The listing builds one solid part. Answer for the finished solid, in the listing's coordinates (mm). A direction names the side the tool comes from. Round coordinates to 2 decimals unless told otherwise and drop trailing zeros.
(1) Find the intervals of material crossed by probe 1 along Z at (x, y) = (0, 3.5); probe 2 along X at (y, z) = (1.1, 0), in increasing order.
(2) For faces 5 (the face through (27.5, 3.9, -0.1)), 6 (the face through (15.05, 3.17, 23.61)), 7 (the face through (-15.79, 4.71, -20.97)), determine the directions among +Z, -Z, +X, -X, +Y, -Y from which every point of the face is accessible in a straight line to the end or side of a thin tool.
(3) Each of these flat-tipped pins is pushed along its axis until it touches: pin 1 Ø2 at (x, z) = (2, -27) entering from +Y; pin 2 Ø1 at (x, z) = (-17.5, 6.5) entering from +Y; pin 3 Ø1 at (x, y) = (11.5, 4) entering from -Z. Where does it stop, or does it pass through?
(4) The mould has two halves that part along Y. Classify faces 1 (the face through (16, 4, 21)), 2 (the face through (-0.1, 3.9, -27.5)), 3 (the face through (-16, 4, -21)), 4 (the face through (-23.977, 1.146, 1.055)): +Y half, -Y half, draft (parallel to the pull), parting line (faces both ways), or undercut.
Autodesk Inventor part; units mm, degrees
ref_plane "YZ Plane" through (0, 0, 0) normal (1, 0, 0) x (0, 1, 0)
ref_plane "XZ Plane" through (0, 0, 0) normal (0, 1, 0) x (-1, 0, 0)
ref_plane "XY Plane" through (0, 0, 0) normal (0, 0, 1) x (1, 0, 0)
sketch "Sketch1" plane through (0, 0, 0) normal (0, 1, 0) x (-1, 0, 0)
  circle A0 centre (0, 0) radius 28
  dimension "d7" = 56
extrude "Extrusion1" add sketch "Sketch1" along normal blind 0.4
sketch "Sketch2" plane through (0, 0.4, 0) normal (0, 1, 0) x (1, 0, 0)
  circle A0 centre (0, 0) radius 27.25
  circle A1 centre (0, 0) radius 28
  dimension "d4" = 54.5
  dimension "d8" = 56
extrude "Extrusion2" add sketch "Sketch2" along normal blind 5
sketch "Sketch3" plane through (0, 5.4, 0) normal (0, 1, 0) x (1, 0, 0)
  arc A0 (-15.63, 22.3219) -> (-17.149, 21.1772) centre (0, 0) ccw
  line L0 (0, 0) -> (-17.149, 21.1772) construction
  line L1 (0, 0) -> (27.25, 0) construction
  line L2 (0, 0) -> (-15.63, 22.3219) construction
  arc A1 (-15.0564, 21.5027) -> (-16.5197, 20.4001) centre (0, 0) ccw
  line L3 (0, 0) -> (-16.5197, 20.4001) construction
  line L4 (0, 0) -> (26.25, 0) construction
  line L5 (0, 0) -> (-15.0564, 21.5027) construction
  line L6 (-16.5197, 20.4001) -> (-17.149, 21.1772)
  line L7 (-15.0564, 21.5027) -> (-15.63, 22.3219)
  circle A2 centre (0, 0) radius 27.25
  dimension "d9" = 27.25
  dimension "d10" = 129
  dimension "d11" = 4
  dimension "d12" = 26.25
  dimension "d13" = 129
  dimension "d14" = 4
extrude "Extrusion3" add sketch "Sketch3" against normal blind 1.4 contours L7 A1 L6 A0
fillet "Fillet1" radius 0.5 4 edges at (-15.3432, 4, -21.9123) (-15.3432, 5.4, -21.9123) (-16.8343, 5.4, -20.7887) (-16.8343, 4, -20.7887)
pattern_circular "Circular Pattern1" count 2 over 360 about axis through (0, 0, 0) along (0, 1, 0) of "Extrusion3", "Fillet1"
sketch "Sketch4" plane through (0, 5.4, 0) normal (0, 1, 0) x (1, 0, 0)
  circle A0 centre (0, 0) radius 28
  line L0 (0, 28) -> (-7.5, 28)
  line L1 (-7.5, 28) -> (-7.5, 25)
  line L2 (-7.5, 25) -> (0, 25)
  line L3 (0, 25) -> (0, 28)
  line L4 (0, 25) -> (7.5, 25)
  line L5 (7.5, 25) -> (7.5, 28)
  line L6 (7.5, 28) -> (0, 28)
  line L7 (0, 28) -> (0, 25)
  circle A1 centre (0, 0) radius 28
  line L8 (28, 0) -> (25, 0)
  line L9 (25, 0) -> (25, 7.5)
  line L10 (25, 7.5) -> (28, 7.5)
  line L11 (28, 7.5) -> (28, 0)
  line L12 (28, 0) -> (25, 0)
  line L13 (25, 0) -> (25, -7.5)
  line L14 (25, -7.5) -> (28, -7.5)
  line L15 (28, -7.5) -> (28, 0)
  dimension "d25" = 7.5
  dimension "d26" = 3
  dimension "d27" = 7.5
  dimension "d28" = 3
  dimension "d51" = 3
  dimension "d52" = 7.5
  dimension "d53" = 3
  dimension "d54" = 7.5
extrude "Extrusion4" cut sketch "Sketch4" against normal blind 1.5 contours L8 L9 L10 A0 | L15 L14 A0 | A0 L14 L13 L8 | A0 L10 L11 | L5 L4 L3 A0 | A0 L6 L5 | L1 L0 A0 | A0 L3 L2 L1
sketch "Sketch7" plane through (0, 0.4, 0) normal (0, 1, 0) x (1, 0, 0)
  circle A0 centre (0, 0) radius 24
  circle A1 centre (0, 0) radius 27.25
  dimension "d47" = 48
  dimension "d50" = 54.5
extrude "Extrusion7" add sketch "Sketch7" along normal blind 1.5
fillet "Fillet5" radius 1 1 edges at (28, 0, 0)
fillet "Fillet5" radius 0.5 2 edges at (-24, 0.4, 0) (-24, 1.9, 0)
properties part number "Diffuser_V1"
Solutions:
1. probe 1: z = -28 to -27.25, 27.25 to 28
1. probe 2: x = -28 to -24, 24 to 28
2. face 5: +X, +Y
2. face 6: +Y, -Y
2. face 7: +Y
3. pin 1: stops at y = 3.9
3. pin 2: stops at y = 0.4
3. pin 3: stops at z = -25.75
4. face 1: undercut
4. face 2: +Y half
4. face 3: undercut
4. face 4: draft
